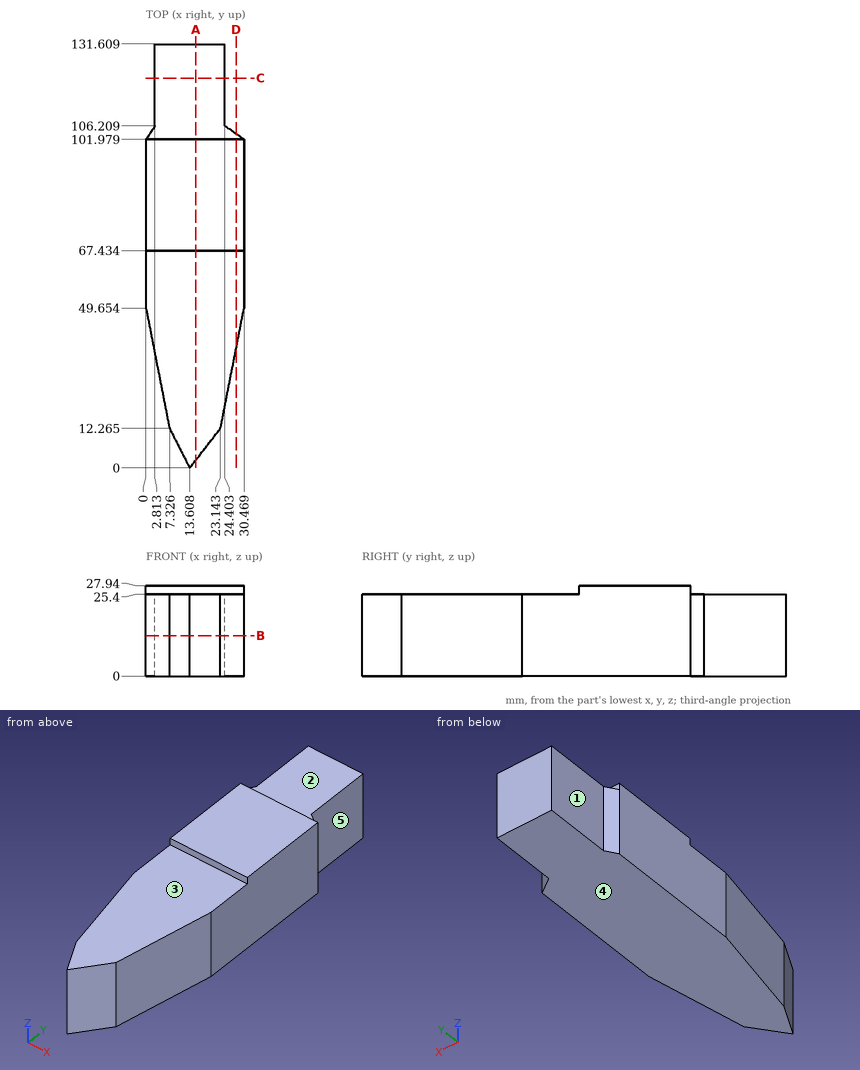
Geometry: see drawing. Coordinates: mm, zero at the bounding-box minimum. A direction names the side the tool comes from. Coordinates: 2 decimals unless noted, no trailing zeros. Loops run counter-clockwise (first coordinate to the right, second up) from the corner with the lowest first, then second, coordinate; pieces in that order, holes last.
(1) Section B-B on z = 12.5. Return the cut outline in (x, y) (1 decimal).
(2) First-contact query: pin 1 Ø1.5 at (x, y) = (5, 104.5) entering from +Z; pin 2 Ø2 at (y, z) = (15, 25) entering from -X (1 decimal); pin 3 Ø12.5 at (y, z) = (115.5, 17.5) entering from +X. Flat tips, straight axial feed; report the tip coordinate or a pass-through.
(3) Section D-D on x = 28. Return the cut outline in (y, z) (1 decimal).
(4) Section C-C on y = 121. Return the cut outline in (x, z).
(5) Section A-A on x = 15.5. Return the cut outline in (y, z) (1 decimal).
(6) Material intervals for probe 1 along X at (y, z) = (107, 13.25); probe 2 along Z at (x, y) = (3.5, 120); probe 3 along Y at (x, z) = (19, 23.25) (1 decimal), sorted ascending.
(7) Set-up query: the marked faces 1, 2, 3, 4 and 5. Return all of +Z, -Z, +X, -X, +Y, -Y with unobstructed straight access to the full face (end or side cutting, diameter ignored); none if empty.
Data:
1. outline: (0, 49.7) - (7.3, 12.3) - (13.6, 0) - (23.1, 12.3) - (30.5, 49.7) - (30.5, 102) - (24.4, 106.2) - (24.4, 131.6) - (2.8, 131.6) - (2.8, 106.2) - (0, 102) - close
2. pin 1: stops at z = 25.4
2. pin 2: stops at x = 6.6
2. pin 3: stops at x = 24.4
3. outline: (37.1, 0) - (103.7, 0) - (103.7, 25.4) - (102, 25.4) - (102, 27.9) - (67.4, 27.9) - (67.4, 25.4) - (37.1, 25.4) - close
4. outline: (2.81, 0) - (24.4, 0) - (24.4, 25.4) - (2.81, 25.4) - close
5. outline: (2.4, 0) - (131.6, 0) - (131.6, 25.4) - (102, 25.4) - (102, 27.9) - (67.4, 27.9) - (67.4, 25.4) - (2.4, 25.4) - close
6. probe 1: x = 2.81 to 24.4
6. probe 2: z = 0 to 25.4
6. probe 3: y = 6.9 to 131.6
7. face 1: +Z, -Z, -X, +Y
7. face 2: +Z, +X, -X, +Y
7. face 3: +Z, +X, -X, -Y
7. face 4: -Z, +X, -X, +Y, -Y
7. face 5: +Z, -Z, +X, +Y
